Could you check a few things on this model? Use its own coordinates, in mm. Face numbers are marked on the shaded views. A direction names the side the tool comes from. Coordinates: 2 decimals unless noted, no trailing zeros. Write each loop counter-clockwise with the first axis right and the second up, starting at its lowest first coordinate (ties: lowest second). Pieces come first, ordered by that corner, then holes.
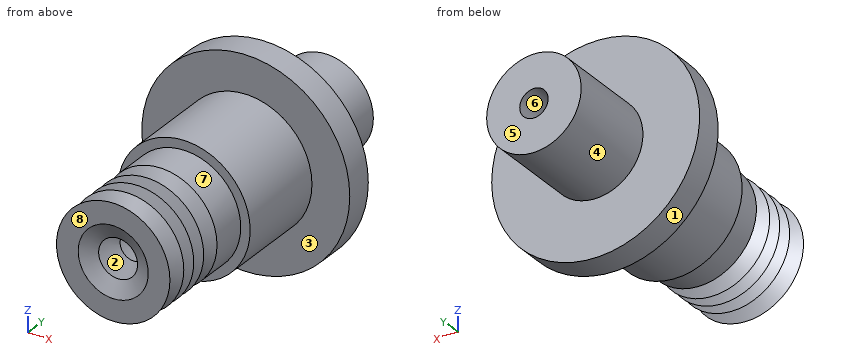
```python
from build123d import *

# Parameters (mm, degrees)
SKETCH_2_R      = 7
EXTRUDE_1_DEPTH = 10
SKETCH_3_R      = 11
EXTRUDE_2_DEPTH = 3
SKETCH_4_R      = 5
SKETCH_4_R_2    = 1.5
EXTRUDE_3_DEPTH = 10


with BuildPart() as part:
    # 草图1 → 旋转1 (revolve)
    with BuildSketch(Plane(origin=(0, 0, 0), x_dir=(-1, 0, 0), z_dir=(0, 0, -1))):
        Polygon((-6, -4), (-3.705599294, -4), (-2.060062716, -3.203134621), (-3.998627726, -1.898006037), (-1.452745067, -0.665140249), (-3.391310077, 0.008460706), (-1.452745067, 0.947227648), (-3.391310077, 1.620828604), (-2.001444472, 2.293883094), (-5, 4.178313324), (-5, 6.465133326), (-2, 6.465133326), (-2, 7.465133326), (-6, 7.465133326), (-6, 3.625681691), (-4.06143499, 2.407398263), (-6, 1.468631321), (-4.06143499, 0.795030366), (-6, -0.143736577), (-4.06143499, -0.817337532), (-6, -1.756104474), (-4.06143499, -3.061233058), align=None)
    revolve(axis=Axis((0, -4, 0), (0, 1, 0)))

    # 草图2 → 凸台-拉伸1 (add)
    with BuildSketch(Plane(origin=(0, 7.465133326, 0), x_dir=(1, 0, 0), z_dir=(0, 1, 0))):
        Circle(SKETCH_2_R)
    extrude(amount=EXTRUDE_1_DEPTH)

    # 草图3 → 凸台-拉伸2 (add)
    with BuildSketch(Plane(origin=(0, 17.465133326, 0), x_dir=(1, 0, 0), z_dir=(0, 1, 0))):
        Circle(SKETCH_3_R)
    extrude(amount=EXTRUDE_2_DEPTH)

    # 草图4 → 凸台-拉伸3 (add)
    with BuildSketch(Plane(origin=(0, 20.465133326, 0), x_dir=(1, 0, 0), z_dir=(0, 1, 0))):
        Circle(SKETCH_4_R)
        Circle(SKETCH_4_R_2, mode=Mode.SUBTRACT)
    extrude(amount=EXTRUDE_3_DEPTH)


solid = part.part
```
1. If we mould it in two halves opening along Z, with no side actions, what happens to the marked faces 6, 7 and 8? For each: pulls with the +Z half, pulls with the -Z half, needs draft (parallel to the pull), parting line crosses it, or undercut.
Verdict:
face 6: undercut
face 7: parting line crosses it
face 8: needs draft
2. For pin 1 (6 mm diameter, centred on y = 1, z = 0, fed in from +X); pin 2 (6 mm diameter, centred on y = 11.5, z = 4, fed in from +X); pin 3 (12 mm diameter, centred on y = 20, z = 7, fed in from -X), each with a flat end and sliding along its axis, tell me the tip position at first contact or that it passes through.
Verdict:
pin 1: stops at x = 6
pin 2: stops at x = 6.93
pin 3: stops at x = -10.95
3. On a 3-axis mill with a long thin cutter (end or side, diameter ignored), from which of +Z, -Z, +X, -X, +Y, -Y can I reach the whole of each face in a straight line? I mean the marked faces 1, 2, 3, 4 and 5. Say none if no direction works.
Verdict:
face 1: +Y, -Y
face 2: none
face 3: -Y
face 4: +Y
face 5: +Z, -Z, +X, -X, +Y
4. I want a section at C-C on z = -2.5. Give the number of separate pieces and of enclosed holes in the cut face, plus the area to 3 significant figures.
Verdict:
separate pieces: 1
enclosed holes: 4
area: 348 mm2
5. I want a section at B-B on y = 9. Please give me the cut outline in (x, z).
Verdict:
outline: circle Ø14 at (0, 0)
6. Please list where these lines run through material, in increasing order: line 1 along X through (y, z) = (5.2, 0); line 2 along X through (y, z) = (25, 0).
Verdict:
line 1: x = -6 to -5, 5 to 6
line 2: x = -5 to -1.5, 1.5 to 5
7. I want a section at A-A on y = 23. Please give me the cut outline in (x, z), plus the area to 3 significant figures.
Verdict:
outline: circle Ø10 at (0, 0); hole circle Ø3 at (0, 0)
area: 71.5 mm2
